The listing builds one solid part. Answer for the finished solid, in the listing's coordinates (mm). Give positions to 0.01 mm unless a question says otherwise; leave off trailing zeros. Write each loop counter-clockwise with the first axis right and the second up, starting at its lowest first coordinate (ties: lowest second). Pieces come first, ordered by that corner, then holes. Notation, with made-up numbers: (-12.75, 42.25) -> (-4.75, 42.25) arc R15 cw to (-4.75, 65.25) -> close; hole circle Ø1 at (68, 25). An arc over 180 degrees is marked (long way). Write each question's results on one line, items separated by ' | '. Start each with the question number.
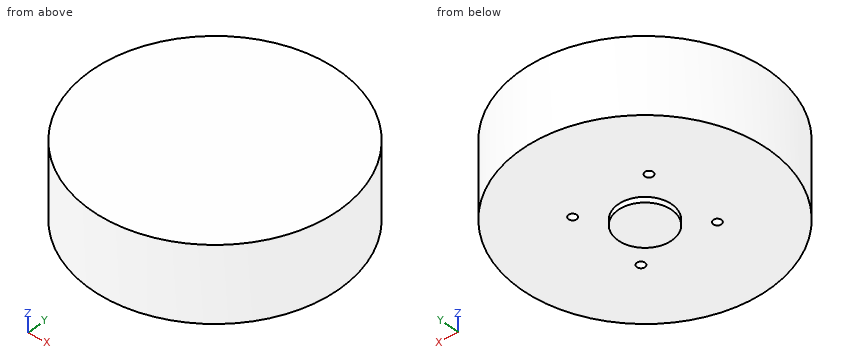
from build123d import *

# Parameters (mm, degrees)
SKETCH1_R           = 46
BOSS_EXTRUDE1_DEPTH = 28
SKETCH4_R           = 1.5
CUT_EXTRUDE1_DEPTH  = 5
SKETCH2_R           = 10
BOSS_EXTRUDE2_DEPTH = 2


with BuildPart() as part:
    # Sketch1 → Boss-Extrude1 (new body)
    with BuildSketch(Plane.XY):
        Circle(SKETCH1_R)
    extrude(amount=BOSS_EXTRUDE1_DEPTH)

    # Sketch4 → Cut-Extrude1 (cut)
    with BuildSketch(Plane(origin=(0, 0, 0), x_dir=(-1, 0, 0), z_dir=(0, 0, -1))):
        with Locations((-14.142135624, 14.142135624)):
            Circle(SKETCH4_R)
        with Locations((14.142135624, 14.142135624)):
            Circle(SKETCH4_R)
        with Locations((-14.142135624, -14.142135624)):
            Circle(SKETCH4_R)
        with Locations((14.142135624, -14.142135624)):
            Circle(SKETCH4_R)
    extrude(amount=-CUT_EXTRUDE1_DEPTH, mode=Mode.SUBTRACT)

    # Sketch2 → Boss-Extrude2 (add)
    with BuildSketch(Plane(origin=(0, 0, 0), x_dir=(-1, 0, 0), z_dir=(0, 0, -1))):
        with Locations(Location((0, 0, 0), (0, 0, 180))):
            Circle(SKETCH2_R)
    extrude(amount=BOSS_EXTRUDE2_DEPTH)


solid = part.part
1. Section A-A (y = 0) is taken. Write down the section's boundary in (x, z), then the cut area to 3 significant figures.
2. Section C-C (z = 24.5) is taken. Write down the section's boundary in (x, y), then the cut area to 3 significant figures.
3. Section D-D (y = 23) is taken. Write down the section's boundary in (x, z), then the cut area to 3 significant figures.
4. Each of these flat-tipped pins is pushed along its axis until it touches: pin 1 Ø12 at (x, z) = (5.5, 7) entering from -Y; pin 2 Ø3.5 at (x, y) = (13.5, -14.5) entering from -Z; pin 3 Ø8 at (y, z) = (23, 24) entering from +X. Where does it stop, or does it pass through?
5. Consider probe 1 along Z at (x, y) = (-28.5, -32.5); probe 2 along X at (y, z) = (-2.5, 6.5); probe 3 along Y at (x, z) = (-37, 22.25). Determine where each line is inside the solid, lowest interval first. Write a range as [from, to].
Results:
1) outline: (-46, 0) -> (-10, 0) -> (-10, -2) -> (10, -2) -> (10, 0) -> (46, 0) -> (46, 28) -> (-46, 28) -> close | area: 2,620 mm²
2) outline: circle Ø92 at (0, 0) | area: 6,650 mm²
3) outline: (-39.84, 0) -> (39.84, 0) -> (39.84, 28) -> (-39.84, 28) -> close | area: 2,230 mm²
4) pin 1: stops at y = -46 | pin 2: stops at z = 0 | pin 3: stops at x = 41.89
5) probe 1: z = [0, 28] | probe 2: x = [-45.93, 45.93] | probe 3: y = [-27.33, 27.33]
